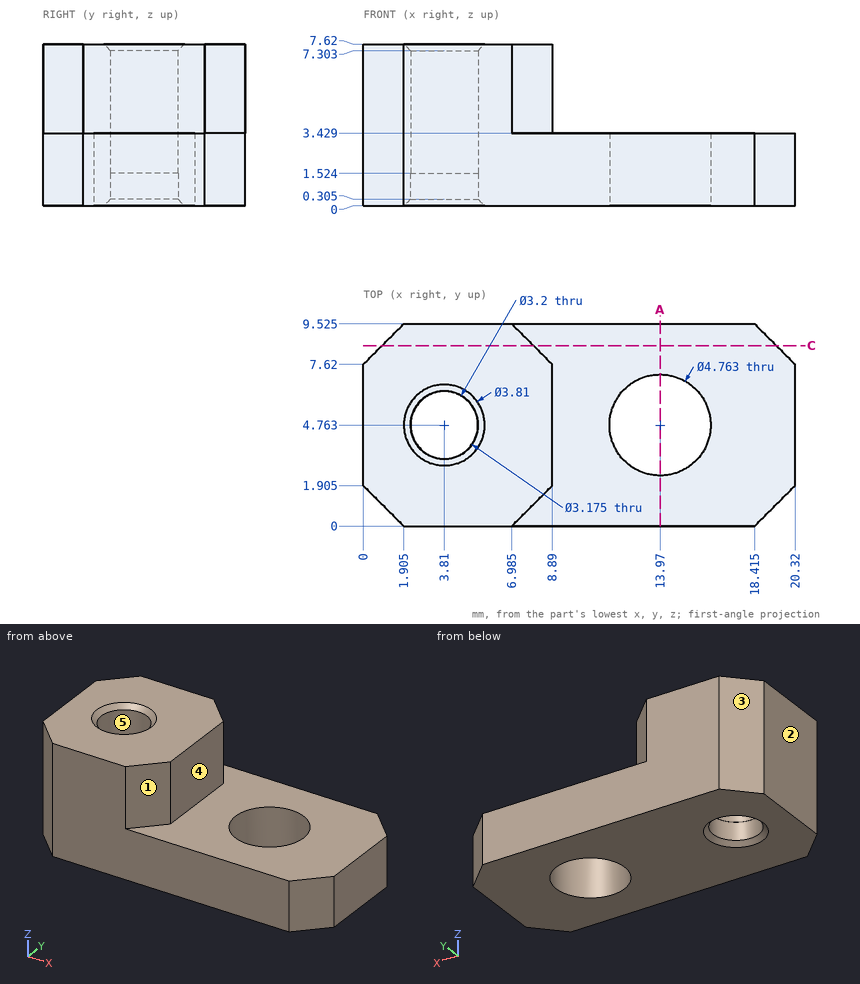
Geometry check sheet. Reference: drawing and pictorial views, mm from the part's lowest x, y, z. A direction names the side the tool comes from. Coordinates: 2 decimals unless noted, no trailing zeros. Order: outer loops, then holes, each group sorted by start corner. A loop starts at its lowest first (then second) coordinate and runs counter-clockwise, first axis right, second up. Notation, with made-up numbers: (61, 64.25) -> (102, 64.25) arc R11 ccw to (102, 83.25) -> close; hole circle Ø8 at (51, 60.5). An arc over 180 degrees is marked (long way). Use CSV: the item, a comma, the result in double quotes. Start each with the question number.
Q1. Section check A-A, the plane x = 13.97. Record the cut outline in (y, z) (1 decimal).
Q2. Tool access check on the marked faces 1 and 2. Record the directions out of +Z, -Z, +X, -X, +Y, -Y that give a thin tool (end or side, any length) a straight path to the whole face; none if there is none.
Q3. Section check C-C, the plane y = 8.5. Record the cut outline in (x, z).
Q4. Thickness scan on line 1 along X through (y, z) = (6, 2.75) (1 decimal); line 2 along X through (y, z) = (5, 1.75); line 3 along Y through (x, z) = (13.97, 2.35) (1 decimal). Record the ranges inside material, lowest first.
Q5. Depth check by flat-ended pin: P1, Ø3.5, axis at x = 3.81, y = 4.76, coming from the -Z side; P2, Ø3, axis at x = 13.97, y = 4.76, coming from the +Z side; P3, Ø3.5, axis at x = 3.5, y = 4.5, coming from the -Z side; P4, Ø2, axis at y = 3.5, z = 5.5, coming from the +X side. Enter the tip coordinate at first touch or a pass-through.
Q6. Draft check along Y on the marked faces 3, 4 and 5. Enter one of: +Y half, -Y half, draft (parallel to the pull), parting line (faces both ways), or undercut.
Returned:
1,outline,"(0, 0) -> (2.4, 0) -> (2.4, 3.4) -> (0, 3.4) -> close; (7.1, 0) -> (9.5, 0) -> (9.5, 3.4) -> (7.1, 3.4) -> close"
2,face 1,"+Z, +X, -Y"
2,face 2,"+Z, -Z, -X, +Y, -Y"
3,outline,"(0.88, 0) -> (19.44, 0) -> (19.44, 3.43) -> (8.01, 3.43) -> (8.01, 7.62) -> (0.88, 7.62) -> close"
4,line 1,"x = 0 to 2.8, 4.8 to 11.9, 16 to 20.3"
4,line 2,"x = 0 to 2.24, 5.38 to 11.6, 16.34 to 20.32"
4,line 3,"y = 0 to 2.4, 7.1 to 9.5"
5,P1,"stops at z = 0.15"
5,P2,"passes through"
5,P3,"stops at z = 0"
5,P4,"stops at x = 8.89"
6,face 3,"+Y half"
6,face 4,"draft"
6,face 5,"undercut"
